```python
from build123d import *

# Parameters (mm, degrees)
F0_W     = 3
F0_H     = 6.8
F1_DEPTH = 12
F2_DEPTH = 5
F3_DEPTH = 3
F0_R     = 6.5
F4_DEPTH = 5
F5_DEPTH = 3
F7_DEPTH = 25
F8_DEPTH = 25
F9_DEPTH = 3


with BuildPart() as f1:
    # F0 (on Top) → F1 (new body)
    with BuildSketch(Plane.XY):
        with Locations((20.2, 23.6)):
            Rectangle(F0_W, F0_H)
        with BuildLine():
            Line((18.7, 20.2), (18.7, 7.6387171698))
            ThreePointArc((18.7, 7.6387171698), (19.8214530244, 3.8923000912), (20.2, 0))
            Line((20.2, 0), (21.7, 0))
            Line((21.7, 0), (21.7, 20.2))
            Line((21.7, 20.2), (18.7, 20.2))
        make_face()
        with BuildLine():
            Line((21.7, 0), (20.2, 0))
            ThreePointArc((20.2, 0), (19.8214530244, -3.8923000912), (18.7, -7.6387171698))
            Line((18.7, -7.6387171698), (18.7, -20.2))
            Line((18.7, -20.2), (21.7, -20.2))
            Line((21.7, -20.2), (21.7, 0))
        make_face()
        with Locations((20.2, -23.6)):
            Rectangle(F0_W, F0_H)
        with BuildLine():
            ThreePointArc((20.2, 0), (19.8214530244, 3.8923000912), (18.7, 7.6387171698))
            Line((18.7, 7.6387171698), (18.7, 0))
            Line((18.7, 0), (20.2, 0))
        make_face()
        with BuildLine():
            ThreePointArc((18.7, -7.6387171698), (19.8214530244, -3.8923000912), (20.2, 0))
            Line((20.2, 0), (18.7, 0))
            Line((18.7, 0), (18.7, -7.6387171698))
        make_face()
    extrude(amount=F1_DEPTH)

    # F0 (on Top) → F2 (join)
    with BuildSketch(Plane.XY):
        with BuildLine():
            Line((0, 18.2), (0, 20.2))
            ThreePointArc((0, 20.2), (-14.28355698, 14.28355698), (-20.2, 0))
            Line((-20.2, 0), (-17.4867563263, -10.1120400111))
            ThreePointArc((-17.4867563263, -10.1120400111), (-11.2572434768, -16.7724318244), (-2.7332534209, -20.0142280825))
            ThreePointArc((-2.7332534209, -20.0142280825), (-1.4686306009, -20.0267809208), (-0.215705511, -20.1988482625))
            ThreePointArc((-0.215705511, -20.1988482625), (-0.1078542929, -20.1997120636), (0, -20.2))
            Line((0, -20.2), (0, -18.2))
            ThreePointArc((0, -18.2), (-18.2, 0), (0, 18.2))
        make_face()
        with BuildLine():
            ThreePointArc((18.7, 7.6387171698), (11.2636120576, 16.7681556355), (0, 20.2))
            Line((0, 20.2), (0, 18.2))
            ThreePointArc((0, 18.2), (12.8693434176, 12.8693434176), (18.2, 0))
            ThreePointArc((18.2, 0), (12.8693434176, -12.8693434176), (0, -18.2))
            Line((0, -18.2), (0, -20.2))
            ThreePointArc((0, -20.2), (11.2636120576, -16.7681556355), (18.7, -7.6387171698))
            Line((18.7, -7.6387171698), (18.7, 0))
            Line((18.7, 0), (18.7, 7.6387171698))
        make_face()
        with BuildLine():
            Line((-17.4867563263, -10.1120400111), (-20.2, 0))
            ThreePointArc((-20.2, 0), (-19.5099010478, -5.23486018), (-17.4867563263, -10.1120400111))
        make_face()
    extrude(amount=F2_DEPTH)

    # F0 (on Top) → F3 (join)
    with BuildSketch(Plane.XY):
        with BuildLine():
            Line((0, 8.8388347648), (0, 18.2))
            ThreePointArc((0, 18.2), (-18.2, 0), (0, -18.2))
            Line((0, -18.2), (0, -8.8388347648))
            Line((0, -8.8388347648), (-7.3388347648, -8.8388347648))
            ThreePointArc((-7.3388347648, -8.8388347648), (-9.8994949366, -9.8994949366), (-8.8388347648, -7.3388347648))
            Line((-8.8388347648, -7.3388347648), (-8.8388347648, 7.3388347648))
            ThreePointArc((-8.8388347648, 7.3388347648), (-9.8994949366, 9.8994949366), (-7.3388347648, 8.8388347648))
            Line((-7.3388347648, 8.8388347648), (0, 8.8388347648))
        make_face()
        with BuildLine():
            Line((7.3388347648, 8.8388347648), (0, 8.8388347648))
            Line((0, 8.8388347648), (0, 5.8))
            ThreePointArc((0, 5.8), (4.1012193309, 4.1012193309), (5.8, 0))
            ThreePointArc((5.8, 0), (4.1012193309, -4.1012193309), (0, -5.8))
            Line((0, -5.8), (0, -8.8388347648))
            Line((0, -8.8388347648), (7.3388347648, -8.8388347648))
            ThreePointArc((7.3388347648, -8.8388347648), (7.7781745931, -7.7781745931), (8.8388347648, -7.3388347648))
            Line((8.8388347648, -7.3388347648), (8.8388347648, 7.3388347648))
            ThreePointArc((8.8388347648, 7.3388347648), (7.7781745931, 7.7781745931), (7.3388347648, 8.8388347648))
        make_face()
        with BuildLine():
            Line((0, 5.8), (0, 8.8388347648))
            Line((0, 8.8388347648), (-7.3388347648, 8.8388347648))
            ThreePointArc((-7.3388347648, 8.8388347648), (-7.7781745931, 7.7781745931), (-8.8388347648, 7.3388347648))
            Line((-8.8388347648, 7.3388347648), (-8.8388347648, -7.3388347648))
            ThreePointArc((-8.8388347648, -7.3388347648), (-7.7781745931, -7.7781745931), (-7.3388347648, -8.8388347648))
            Line((-7.3388347648, -8.8388347648), (0, -8.8388347648))
            Line((0, -8.8388347648), (0, -5.8))
            ThreePointArc((0, -5.8), (-5.8, 0), (0, 5.8))
        make_face()
        with BuildLine():
            ThreePointArc((18.2, 0), (12.8693434176, 12.8693434176), (0, 18.2))
            Line((0, 18.2), (0, 8.8388347648))
            Line((0, 8.8388347648), (7.3388347648, 8.8388347648))
            ThreePointArc((7.3388347648, 8.8388347648), (8.8388347648, 10.3388347648), (10.3388347648, 8.8388347648))
            ThreePointArc((10.3388347648, 8.8388347648), (9.8994949366, 7.7781745931), (8.8388347648, 7.3388347648))
            Line((8.8388347648, 7.3388347648), (8.8388347648, -7.3388347648))
            ThreePointArc((8.8388347648, -7.3388347648), (9.8994949366, -7.7781745931), (10.3388347648, -8.8388347648))
            ThreePointArc((10.3388347648, -8.8388347648), (8.8388347648, -10.3388347648), (7.3388347648, -8.8388347648))
            Line((7.3388347648, -8.8388347648), (0, -8.8388347648))
            Line((0, -8.8388347648), (0, -18.2))
            ThreePointArc((0, -18.2), (12.8693434176, -12.8693434176), (18.2, 0))
        make_face()
    extrude(amount=F3_DEPTH)

    # F0 (on Top) → F4 (join)
    with BuildSketch(Plane.XY):
        with BuildLine():
            ThreePointArc((-0.215705511, -20.1988482625), (-1.4686306009, -20.0267809208), (-2.7332534209, -20.0142280825))
            ThreePointArc((-2.7332534209, -20.0142280825), (-1.4773661863, -20.14590254), (-0.215705511, -20.1988482625))
        make_face()
        with BuildLine():
            ThreePointArc((-0.215705511, -20.1988482625), (-1.4773661863, -20.14590254), (-2.7332534209, -20.0142280825))
            ThreePointArc((-2.7332534209, -20.0142280825), (-9.3953899149, -23.0554795722), (-12.1984032717, -29.8213046815))
            ThreePointArc((-12.1984032717, -29.8213046815), (-2.2893512261, -39.99960081), (7.8, -30))
            ThreePointArc((7.8, -30), (5.5408961009, -23.6692395753), (-0.215705511, -20.1988482625))
        make_face()
        with Locations((-2.2, -30)):
            Circle(F0_R, mode=Mode.SUBTRACT)
    extrude(amount=F4_DEPTH)

    # F0 (on Top) → F5 (join)
    with BuildSketch(Plane.XY):
        with BuildLine():
            ThreePointArc((-2.7332534209, -20.0142280825), (-11.2572434768, -16.7724318244), (-17.4867563263, -10.1120400111))
            Line((-17.4867563263, -10.1120400111), (-12.1984032717, -29.8213046815))
            ThreePointArc((-12.1984032717, -29.8213046815), (-9.3953899149, -23.0554795722), (-2.7332534209, -20.0142280825))
        make_face()
        with BuildLine():
            Line((18.7, -20.2), (18.7, -7.6387171698))
            ThreePointArc((18.7, -7.6387171698), (11.2636120576, -16.7681556355), (0, -20.2))
            Line((0, -20.2), (18.7, -20.2))
        make_face()
        with BuildLine():
            Line((18.7, -20.2), (0, -20.2))
            ThreePointArc((0, -20.2), (-0.1078542929, -20.1997120636), (-0.215705511, -20.1988482625))
            ThreePointArc((-0.215705511, -20.1988482625), (5.5408961009, -23.6692395753), (7.8, -30))
            Line((7.8, -30), (18.7, -20.2))
        make_face()
    extrude(amount=F5_DEPTH)

    # F6 (on face) → F7 (cut)
    with BuildSketch(Plane(origin=(18.7, 0, 0), x_dir=(0, -1, 0), z_dir=(-1, 0, 0))):
        with BuildLine():
            Line((-25.2, 6), (-23.5, 6))
            Line((-23.5, 6), (-23.5, 7.7))
            ThreePointArc((-23.5, 7.7), (-24.702081528, 7.202081528), (-25.2, 6))
        make_face()
        with BuildLine():
            Line((-21.8, 6), (-23.5, 6))
            Line((-23.5, 6), (-25.2, 6))
            ThreePointArc((-25.2, 6), (-23.5, 4.3), (-21.8, 6))
        make_face()
        with BuildLine():
            Line((-23.5, 7.7), (-23.5, 6))
            Line((-23.5, 6), (-21.8, 6))
            ThreePointArc((-21.8, 6), (-22.297918472, 7.202081528), (-23.5, 7.7))
        make_face()
    extrude(amount=-F7_DEPTH, mode=Mode.SUBTRACT)

    # F6 (on face) → F8 (cut)
    with BuildSketch(Plane(origin=(18.7, 0, 0), x_dir=(0, -1, 0), z_dir=(-1, 0, 0))):
        with BuildLine():
            Line((-21.8, 6), (-23.5, 6))
            Line((-23.5, 6), (-25.2, 6))
            ThreePointArc((-25.2, 6), (-23.5, 4.3), (-21.8, 6))
        make_face()
        with BuildLine():
            Line((-25.2, 6), (-23.5, 6))
            Line((-23.5, 6), (-23.5, 7.7))
            ThreePointArc((-23.5, 7.7), (-24.702081528, 7.202081528), (-25.2, 6))
        make_face()
        with BuildLine():
            Line((-23.5, 7.7), (-23.5, 6))
            Line((-23.5, 6), (-21.8, 6))
            ThreePointArc((-21.8, 6), (-22.297918472, 7.202081528), (-23.5, 7.7))
        make_face()
        with BuildLine():
            ThreePointArc((23.5, 9.2), (22.297918472, 6.297918472), (25.2, 7.5))
            ThreePointArc((25.2, 7.5), (24.702081528, 8.702081528), (23.5, 9.2))
        make_face()
    extrude(amount=-F8_DEPTH, mode=Mode.SUBTRACT)

    # F0 (on Top) → F9 (join)
    with BuildSketch(Plane.XY):
        with BuildLine():
            Line((18.7, 20.2), (0, 20.2))
            ThreePointArc((0, 20.2), (11.2636120576, 16.7681556355), (18.7, 7.6387171698))
            Line((18.7, 7.6387171698), (18.7, 20.2))
        make_face()
    extrude(amount=F9_DEPTH)


with BuildPart() as f10_1:
    # F10: copy of F1
    add(f1.part)


solid = f10_1.part
```
Here's how the part is built. I have some questions about the finished solid (model axes, mm). A direction names the side the tool comes from. Give positions to 0.01 mm unless a question says otherwise; leave off trailing zeros. Write each loop counter-clockwise with the first axis right and the second up, starting at its lowest first coordinate (ties: lowest second). Pieces come first, ordered by that corner, then holes.
(1) Will these pins go through, and if not, where does the flat tip stop? pin 1 (3.5 mm diameter, centred on x = 20.5, z = 7, fed in from -Y); pin 2 (16 mm diameter, centred on x = -10.5, y = -16, fed in from +Z); pin 3 (4 mm diameter, centred on x = 11, y = 11, fed in from +Z).
Output values:
pin 1: stops at y = -27
pin 2: stops at z = 5
pin 3: stops at z = 3
(2) Imagine slicing it at B-B, the plane y = -28.5. Write out the boundary of the cut face in (x, z).
Output values:
outline: (-12.55, 0) - (-8.52, 0) - (-8.52, 5) - (-12.09, 5) - (-12.09, 3) - (-12.55, 3) - close; (4.12, 0) - (9.47, 0) - (9.47, 3) - (7.69, 3) - (7.69, 5) - (4.12, 5) - close
(3) Imagine slicing it at C-C, the plane x = -6.5. Write out the boundary of the cut face in (y, z).
Output values:
outline: (-39.03, 0) - (-34.87, 0) - (-34.87, 5) - (-39.03, 5) - close; (-25.13, 0) - (19.13, 0) - (19.13, 5) - (17, 5) - (17, 3) - (-17, 3) - (-17, 5) - (-19.13, 5) - (-19.13, 3) - (-20.97, 3) - (-20.97, 5) - (-25.13, 5) - close
(4) Thinking about a two-plate mould opening in Y: for faces 4 (the face through (-14.88, -19.83, 1.48)), 5 (the face through (18.7, 0, 7)), 6 (the face through (-12, -20, 3)), which applies, pulls with the +Y half, pulls with the -Y half, needs draft (parallel to the pull), parting line crosses it, or undercut?
Output values:
face 4: pulls with the -Y half
face 5: needs draft
face 6: undercut
(5) Imagine slicing it at A-A, the plane x = 3.5. Write out the boundary of the cut face in (y, z).
Output values:
outline: (-38.22, 0) - (-33.12, 0) - (-33.12, 5) - (-38.22, 5) - close; (-26.88, 0) - (-4.62, 0) - (-4.62, 3) - (-17.86, 3) - (-17.86, 5) - (-19.89, 5) - (-19.89, 3) - (-21.78, 3) - (-21.78, 5) - (-26.88, 5) - close; (4.62, 0) - (20.2, 0) - (20.2, 3) - (19.89, 3) - (19.89, 5) - (17.86, 5) - (17.86, 3) - (4.62, 3) - close
(6) If I drill on L1, parallel to X at y = -25, z = 4; L2, parallel to Y at x = 20.4, z = 7.5; L3, parallel to Y at x = 5.5, z = 3.5, over which ranges is the centre line in solid material (lowest first)?
Output values:
L1: x = -10.86 to -6.35, 1.95 to 6.46, 18.7 to 21.7
L2: y = -27 to -25.2, -21.8 to 22.7, 24.3 to 27
L3: y = -36.38 to -23.62, -19.44 to -17.35, 17.35 to 19.44
(7) Imagine slicing it at D-D, the plane x = -13. Write out the boundary of the cut face in (y, z).
Output values:
outline: (-26.83, 0) - (15.46, 0) - (15.46, 5) - (12.74, 5) - (12.74, 3) - (-12.74, 3) - (-12.74, 5) - (-15.46, 5) - (-15.46, 3) - (-26.83, 3) - close
(8) On a 3-axis mill with a long thin cutter (end or side, diameter ignored), from which of +Z, -Z, +X, -X, +Y, -Y can I reach the whole of each face in a straight line? I mean faces 1 (the face through (14, 16, 3)), 2 (the face through (13.17, -25.17, 1.48)), 3 (the face through (20, -27, 6)). Say none if no direction works.
Output values:
face 1: +Z, +Y
face 2: +Z, -Z, -Y
face 3: +Z, -Z, +X, -Y
